from build123d import *

# Parameters (mm, degrees)
F1_DEPTH = 15
F2_DEPTH = 10
F3_DEPTH = 5


with BuildPart() as f1:
    # F0 (on Top) → F1 (new body)
    with BuildSketch(Plane.XY):
        Polygon((-37.712831, 21.99769), (-45.967648, 21.99769), (-37.712831, -10.45064), (-29.458014, -10.45064), (-25.330606, 5.773525), (-21.203197, -10.45064), (-12.94838, -10.45064), (-4.693563, 21.99769), (-12.94838, 21.99769), (-17.075789, 5.773525), (-21.203197, 21.99769), (-29.458014, 21.99769), (-33.585422, 5.773525), align=None)
    extrude(amount=F1_DEPTH)

    # F0 (on Top) → F2 (join)
    with BuildSketch(Plane.XY):
        with BuildLine():
            Line((-4.693563, 21.99769), (-12.94838, -10.45064))
            Line((-12.94838, -10.45064), (-4.693563, -10.45064))
            Line((-4.693563, -10.45064), (-3.826923, -7.044018))
            Line((-3.826923, -7.044018), (-3.437773, -5.514332))
            Line((-3.437773, -5.514332), (-1.565072, 1.846947))
            Line((-1.565072, 1.846947), (-1.564775, 1.848116))
            ThreePointArc((-1.564775, 1.848116), (11.072878, 9.361753), (3.556356, 21.99769))
            Line((3.556356, 21.99769), (-4.693563, 21.99769))
        make_face()
        with BuildLine():
            ThreePointArc((2.257058, 16.871111), (5.946883, 10.663352), (-0.260876, 6.973526))
            Line((-0.260876, 6.973526), (2.257058, 16.871111))
        make_face(mode=Mode.SUBTRACT)
    extrude(amount=F2_DEPTH)

    # F0 (on Top) → F3 (join)
    with BuildSketch(Plane.XY):
        with BuildLine():
            Line((3.561253, 21.99769), (3.556356, 21.99769))
            ThreePointArc((3.556356, 21.99769), (11.072878, 9.361753), (-1.564775, 1.848116))
            Line((-1.564775, 1.848116), (-1.565072, 1.846947))
            Line((-1.565072, 1.846947), (-3.437773, -5.514332))
            Line((-3.437773, -5.514332), (2.371906, -5.514332))
            Line((2.371906, -5.514332), (2.883339, -3.503974))
            ThreePointArc((2.883339, -3.503974), (16.514622, 11.049437), (4.60158, 27.039842))
            Line((4.60158, 27.039842), (3.561253, 21.99769))
        make_face()
        Polygon((-3.826923, -7.044018), (-4.693563, -10.45064), (1.116115, -10.45064), (1.982756, -7.044018), align=None)
    extrude(amount=F3_DEPTH)


solid = f1.part
Can you work these out from the model? Positions are in its coordinate system, mm. A direction names the side the tool comes from. Give positions to 0.01 mm unless a question says otherwise; leave off trailing zeros. Loops run counter-clockwise (first coordinate to the right, second up) from the corner with the lowest first, then second, coordinate; pieces in that order, holes last. Notation, with made-up numbers: M 28.25,-14.5 L 41.25,-14.5 A21 ccw 41.25,-9.5 Z; hole C -16,-11.75 d3. An arc over 180 degrees is marked long. One line per item, written item: value. Start each with the question number.
1) Thinking about a two-plate mould opening in X: for faces 4 (the face through (-25, 21.998, 7)), 5 (the face through (-31.493, 13.999, 7.395)), 6 (the face through (1.543, -8.771, 2.465)), which applies, +X half, -X half, draft (parallel to the pull), parting line (faces both ways), or undercut?
2) I'm going to push flat-ended pins straight in: pin 1 (1 mm diameter, centred on y = 15.5, z = 2, fed in from +X); pin 2 (5 mm diameter, centred on y = 16.5, z = 7.5, fed in from -X); pin 3 (6 mm diameter, centred on y = 13, z = 13, fed in from -X). Where does each tip first touch, or does it pass through?
3) On a 3-axis mill with a long thin cutter (end or side, diameter ignored), from which of +Z, -Z, +X, -X, +Y, -Y can I reach the whole of each face in a straight line? I mean faces 1 (the face through (-19.11, 13.77, 7.4)), 2 (the face through (-8.879, 5.546, 12.465)), 3 (the face through (-23.296, -2.225, 7.395)). Say none if no direction works.
4) If we section it at C-C, the plane z = 10.75: Write out the boundary of the cut face in (x, y).
5) If I drill on line 1 (X direction, y = 9, z = 7); line 2 (X direction, y = 14.5, z = 3); line 3 (X direction, y = 15.5, z = 13.5), over which ranges is the centre line in solid material (lowest first)? Write a range as [from, to].
6) If we section it at D-D, the plane y = 14.5: Write out the boundary of the cut face in (x, z).
7) If we section it at A-A, the plane z = 1.5: Write out the boundary of the cut face in (x, y), and give its area (3 significant figures).
8) If we section it at B-B, the plane y = -4.5: Write out the boundary of the cut face in (x, z).
Completed:
1. face 4: draft
1. face 5: undercut
1. face 6: +X half
2. pin 1: stops at x = 16.23
2. pin 2: stops at x = -45.21
2. pin 3: stops at x = -44.44
3. face 1: +Z, -Z, +Y
3. face 2: +Z, +X, -Y
3. face 3: +Z, -Z, -Y
4. outline: M -45.97,22 L -37.71,-10.45 L -29.46,-10.45 L -25.33,5.77 L -21.2,-10.45 L -12.95,-10.45 L -4.69,22 L -12.95,22 L -17.08,5.77 L -21.2,22 L -29.46,22 L -33.59,5.77 L -37.71,22 Z
5. line 1: x = [-42.66, -34.41], [-32.76, -17.9], [-16.25, 0.25], [5.19, 10.97]
5. line 2: x = [-44.06, -35.81], [-31.37, -19.3], [-14.86, 1.65], [5.41, 16.32]
5. line 3: x = [-44.31, -36.06], [-31.11, -19.55], [-14.6, -6.35]
6. outline: M -44.06,0 L -35.81,0 L -35.81,15 L -44.06,15 Z; M -31.37,0 L -19.3,0 L -19.3,15 L -31.37,15 Z; M -14.86,0 L 1.65,0 L 1.65,10 L -6.6,10 L -6.6,15 L -14.86,15 Z; M 5.41,0 L 16.32,0 L 16.32,5 L 11.07,5 L 11.07,10 L 5.41,10 Z
7. outline: M -45.97,22 L -37.71,-10.45 L -29.46,-10.45 L -25.33,5.77 L -21.2,-10.45 L 1.12,-10.45 L 1.98,-7.04 L -3.83,-7.04 L -3.44,-5.51 L 2.37,-5.51 L 2.88,-3.5 A15.54 ccw 4.6,27.04 L 3.56,22 L -12.95,22 L -17.08,5.77 L -21.2,22 L -29.46,22 L -33.59,5.77 L -37.71,22 Z; hole M -0.26,6.97 A5.11 ccw 2.26,16.87 Z
7. area: 1,510 mm^2
8. outline: M -39.23,0 L -27.94,0 L -27.94,15 L -39.23,15 Z; M -22.72,0 L 2.63,0 L 2.63,5 L -3.18,5 L -3.18,10 L -11.43,10 L -11.43,15 L -22.72,15 Z
